Geometry check sheet. Reference: the model listing, model coordinates, mm. Face numbers are marked on the shaded views. A direction names the side the tool comes from. Give positions to 0.01 mm unless a question says otherwise; leave off trailing zeros. Write each loop counter-clockwise with the first axis right and the second up, starting at its lowest first coordinate (ties: lowest second). Pieces come first, ordered by that corner, then holes. Notation, with made-up numbers: M 14.5,28.5 L 50.5,28.5 A25 cw 50.5,62.5 Z; hole C -29,-0.75 d4. An arc over 180 degrees is marked long. Write each question's results on one line, items separated by ' | '.
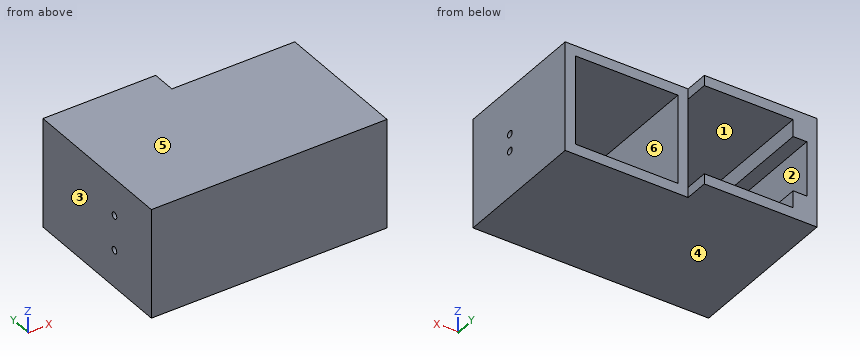
Autodesk Inventor part; units mm, degrees
ref_plane "YZ Plane" through (0, 0, 0) normal (1, 0, 0) x (0, 1, 0)
ref_plane "XZ Plane" through (0, 0, 0) normal (0, 1, 0) x (-1, 0, 0)
ref_plane "XY Plane" through (0, 0, 0) normal (0, 0, 1) x (1, 0, 0)
sketch "Esboço1" plane through (0, 0, 0) normal (0, 1, 0) x (-1, 0, 0)
  line L0 (0, 0) -> (0, -16)
  line L1 (0, -16) -> (-34.5, -16)
  line L2 (-34.5, -16) -> (-34.5, 0)
  line L3 (-34.5, 0) -> (0, 0)
  line L4 (-3.5, -14.5) -> (-16.5, -14.5)
  line L5 (-16.5, -14.5) -> (-16.5, -1.5)
  line L6 (-16.5, -1.5) -> (-3.5, -1.5)
  line L7 (-18, -14.5) -> (-33, -14.5)
  line L8 (-33, -14.5) -> (-33, -1.5)
  line L9 (-33, -1.5) -> (-18, -1.5)
  line L10 (-18, -1.5) -> (-18, -14.5)
  line L11 (-3.5, -14.5) -> (-3.5, -12)
  line L12 (-3.5, -12) -> (-1.5, -12)
  line L13 (-1.5, -12) -> (-1.5, -4)
  line L14 (-1.5, -4) -> (-3.5, -4)
  line L15 (-3.5, -4) -> (-3.5, -1.5)
  point P0 (-34.5, -8)
  dimension "d0" = 13
  dimension "d1" = 13
  dimension "d2" = 15
  dimension "d3" = 13
  dimension "d4" = 8
  dimension "d5" = 2.5
  dimension "d6" = 1.5
  dimension "d7" = 1.5
  dimension "d8" = 2
  dimension "d9" = 1.5
  dimension "d10" = 1.5
  dimension "d11" = 1.5
extrude "Extrusão1" add sketch "Esboço1" along normal blind 1.5 contours L4 L5 L6 L15 L14 L13 L12 L11 | L7 L8 L9 L10
extrude "Extrusão2" add sketch "Esboço1" along normal blind 20
sketch "Esboço2" plane through (0, 0, -16) normal (-1, 0, 0) x (0, 0, 1)
  line L0 (12, 20) -> (4, 20)
  line L1 (8, 20) -> (8, 0)
  line L2 (0, 0) -> (0, 20)
  circle A0 centre (5.45, 8) radius 0.5
  circle A1 centre (10.55, 8) radius 0.5
  line L3 (0, 0) -> (16, 0)
  dimension "d23" = 8
extrude "Extrusão3" cut sketch "Esboço2" against normal blind 10
sketch "Esboço3" plane through (34.5, 0, 0) normal (1, 0, 0) x (0, 0, -1)
  line L0 (0, 20) -> (16, 20)
  line L1 (8, 20) -> (8, 0)
  circle A0 centre (6.75, 8) radius 0.5
  circle A1 centre (9.25, 8) radius 0.5
  line L2 (0, 0) -> (16, 0)
  line L3 (11, 16) -> (11, 8)
  line L4 (11, 8) -> (5, 8)
  line L5 (5, 8) -> (5, 16)
  circle A2 centre (5, 12) radius 1.5
  circle A3 centre (11, 12) radius 1.5
  dimension "d26" = 1
  dimension "d27" = 1
  dimension "d28" = 8
  dimension "d29" = 8
  dimension "d30" = 1.25
  dimension "d31" = 1.25
  dimension "d78" = 3
  dimension "d79" = 3
  dimension "d80" = 3
  dimension "d81" = 3
extrude "Extrusão4" cut sketch "Esboço3" against normal blind 10 contours L4 A0 | A1 L4 | L4 A1 | A0 L4
sketch "Esboço4" plane through (18, 1.5, -14.5) normal (1, 0, 0) x (0, 0, -1)
  line L0 (-14.5, -1.5) -> (1.5, -1.5)
  line L1 (-6.5, -1.5) -> (-6.5, 18.5)
  line L2 (0, 18.5) -> (-13, 18.5)
  circle A0 centre (-6.5, 6.5) radius 0.5
  line L3 (0, 0) -> (-13, 0)
  dimension "d40" = 1
  dimension "d42" = 6.5
extrude "Extrusão5" cut sketch "Esboço4" against normal blind 10
sketch "Esboço6" plane through (0, 20, 0) normal (0, 1, 0) x (1, 0, 0)
  line L0 (0, 0) -> (34.5, 0)
  line L1 (0, 0) -> (16.5, 0)
  line L2 (0, 0) -> (16.5, 0) construction
  line L3 (16.5, 14.5) -> (16.5, 1.5)
  line L4 (16.5, 0) -> (16.5, 1.5)
  line L5 (16.5, 1.5) -> (3.5, 1.5)
  line L6 (16.5, 1.5) -> (3.5, 1.5)
  line L7 (3.5, 1.5) -> (3.5, 4)
  line L8 (3.5, 1.5) -> (3.5, 4)
  line L9 (3.5, 4) -> (1.5, 4)
  line L10 (3.5, 4) -> (1.5, 4)
  line L11 (1.5, 4) -> (1.5, 12)
  line L12 (1.5, 12) -> (3.5, 12)
  line L13 (1.5, 12) -> (3.5, 12)
  line L14 (3.5, 12) -> (3.5, 14.5)
  line L15 (3.5, 12) -> (3.5, 14.5)
  line L16 (3.5, 14.5) -> (16.5, 14.5)
  line L17 (3.5, 14.5) -> (16.5, 14.5)
  line L18 (16.5, 14.5) -> (16.5, 16)
  line L19 (34.5, 16) -> (0, 16)
  line L20 (0, 16) -> (0, 0)
  line L21 (0, 16.0004) -> (0, 0)
  dimension "d66" = 16.5
  dimension "d67" = 0
extrude "Extrusão8" add sketch "Esboço6" along normal blind 3.5 contours L20 L19 L18 L16 L14 L12 L11 L9 L7 L5 L4 L0
properties part number "Base_3DPrint"
Q1. Section check D-D (x = 19). Enter the section's corners in (y, z), then the cut area to 3 significant figures.
Answer key:
outline: M 0,-16 L 20,-16 L 20,-14.5 L 1.5,-14.5 L 1.5,-1.5 L 20,-1.5 L 20,0 L 0,0 Z | area: 79.5 mm2
Q2. Material ranges on probe 1 along Z at (x, y) = (33.3, 8); probe 2 along X at (y, z) = (5.5, -9); probe 3 along X at (y, z) = (5, -1.75), recorded low to high. Write a range as [from, to].
Answer key:
probe 1: z = [-16, -9.75], [-8.75, -7.25], [-6.25, 0] | probe 2: x = [0, 1.5], [16.5, 18], [33, 34.5] | probe 3: x = [0, 3.5], [16.5, 18], [33, 34.5]
Q3. Release check for a two-part mould opening along Z. For the marked faces 1, 2, 3 and 4 record: released by +Z, released by -Z, zero draft, split by the parting line, or undercut.
Answer key:
face 1: undercut | face 2: undercut | face 3: zero draft | face 4: released by -Z
Q4. Access from +Z, -Z, +X, -X, +Y, -Y to the whole of each face (thin tool, end or side, straight path). Record for the marked faces 5 and 6.
Answer key:
face 5: +Z, +X, -X, +Y, -Y | face 6: +Y
Q5. Section check B-B (y = 18). Enter the section's corners in (x, z), then the cut area to 3 significant figures.
Answer key:
outline: M 0,-16 L 34.5,-16 L 34.5,0 L 0,0 Z; hole M 1.5,-12 L 3.5,-12 L 3.5,-14.5 L 16.5,-14.5 L 16.5,-1.5 L 3.5,-1.5 L 3.5,-4 L 1.5,-4 Z; hole M 18,-14.5 L 33,-14.5 L 33,-1.5 L 18,-1.5 Z | area: 172 mm2
Q6. Section check A-A (z = -9.25). Enter the section's corners in (x, y).
Answer key:
outline: M 0,0 L 34.5,0 L 34.5,7.5 L 33,7.5 L 33,1.5 L 18,1.5 L 18,20 L 16.5,20 L 16.5,1.5 L 1.5,1.5 L 1.5,23.5 L 0,23.5 Z; M 33,8.5 L 34.5,8.5 L 34.5,20 L 33,20 Z
Q7. Section check C-C (x = 14). Enter the section's corners in (y, z), then the cut area to 3 significant figures.
Answer key:
outline: M 0,-16 L 23.5,-16 L 23.5,-14.5 L 1.5,-14.5 L 1.5,-1.5 L 23.5,-1.5 L 23.5,0 L 0,0 Z | area: 90.0 mm2
Q8. Depth check by flat-ended pin: P1, Ø1.2, axis at y = 22.5, z = -1, coming from the +X side; P2, Ø6.5, axis at x = 10.5, z = -11, coming from the +Y side. Enter the tip coordinate at first touch or a pass-through.
Answer key:
P1: stops at x = 16.5 | P2: stops at y = 1.5
